Autodesk Inventor part; units mm, degrees
ref_plane "YZ Plane" through (0, 0, 0) normal (1, 0, 0) x (0, 1, 0)
ref_plane "XZ Plane" through (0, 0, 0) normal (0, 1, 0) x (-1, 0, 0)
ref_plane "XY Plane" through (0, 0, 0) normal (0, 0, 1) x (1, 0, 0)
sketch "Sketch1" plane through (0, 0, 0) normal (0, 1, 0) x (-1, 0, 0)
  circle A0 centre (0, 0) radius 11
  circle A1 centre (0, 0) radius 12.5
  dimension "d0" = 22
  dimension "d1" = 25
extrude "Extrusion1" add sketch "Sketch1" along normal blind 7
sketch "Sketch2" plane through (0, 7, 0) normal (0, 1, 0) x (1, 0, 0)
  circle A0 centre (0, -18.05) radius 2.15
  circle A1 centre (0, 18.05) radius 2.15
  circle A2 centre (0, -18.05) radius 5.95
  circle A3 centre (0, 18.05) radius 5.95
  line L0 (-5.5444, -20.2091) -> (-11.6479, -4.536)
  line L1 (5.5444, -20.2091) -> (11.6479, -4.536)
  line L2 (-11.6479, 4.536) -> (-5.5444, 20.2091)
  line L3 (11.6479, 4.536) -> (5.5444, 20.2091)
  circle A4 centre (0, 0) radius 12.5
  dimension "d4" = 4.3
  dimension "d5" = 4.3
  dimension "d6" = 0
  dimension "d7" = 0
  dimension "d8" = 18.05
  dimension "d9" = 18.05
  dimension "d10" = 3.8
  dimension "d11" = 3.8
extrude "Extrusion2" add sketch "Sketch2" against normal blind 3.5 contours A2 A4 | L0 A4 A2 | A2 A4 L1 | L2 A3 A4 | A3 A4 | A4 A3 L3 picked at (3.4679, -21.155) picked at (3.4679, 21.155)
properties part number "chumacera"
Design review of the part built by this model. Coordinates are the model's own, in mm. A direction names the side the tool comes from. Coordinates: 2 decimals unless noted, no trailing zeros. Order: outer loops, then holes, each group sorted by start corner. A loop starts at its lowest first (then second) coordinate and runs counter-clockwise, first axis right, second up.
1) Clearance check with flat-ended pins moving along their axes: pin 1 (5.5 mm diameter, centred on x = 0, z = -18.05, fed in from +Y); pin 2 (2.5 mm diameter, centred on x = 0, z = 18.05, fed in from +Y); pin 3 (3 mm diameter, centred on y = 2.5, z = -7.5, fed in from +X); pin 4 (2 mm diameter, centred on y = 1, z = 9, fed in from -X). State where each tip first meets the part, or that it passes through.
2) Take a section at C-C, the plane x = 9.75. Give the boundary of the cut face in (y, z).
3) Wall thickness on line 1 along Z through (x, y) = (0, 4.75); line 2 along Z through (x, y) = (0, 2); line 3 along X through (y, z) = (3.5, -4): over which ranges is each line inside the solid? List them lowest first.
4) Take a section at A-A, the plane x = 0. Give the boundary of the cut face in (y, z).
5) Take a section at D-D, the plane y = 4.5. Give the boundary of the cut face in (x, z).
6) For faces 1 (the flat face through (-8.553, 5.274, 12.482)), 2 (the cylindrical face through (1.627, 2.673, -12.394)), list the 3-axis set-ups (+Z, -Z, +X, -X, +Y, -Y) from which the entire face can be reached by the end or side of a thin tool; tool diameter is ignored.
7) Take a section at B-B, the plane z = -8. Give the boundary of the cut face in (x, y), and give its area (3 significant figures).
Returned:
1. pin 1: stops at y = 7
1. pin 2: passes through
1. pin 3: stops at x = 10.97
1. pin 4: stops at x = -9.6
2. outline: (0, -7.82) - (3.5, -7.82) - (3.5, -9.41) - (7, -9.41) - (7, -5.09) - (0, -5.09) - close; (0, 5.09) - (7, 5.09) - (7, 9.41) - (3.5, 9.41) - (3.5, 7.82) - (0, 7.82) - close
3. line 1: z = -24 to -20.2, -15.9 to -11, 11 to 15.9, 20.2 to 24
3. line 2: z = -12.5 to -11, 11 to 12.5
3. line 3: x = -11.84 to -10.25, 10.25 to 11.84
4. outline: (0, -12.5) - (3.5, -12.5) - (3.5, -15.9) - (7, -15.9) - (7, -11) - (0, -11) - close; (0, 11) - (7, 11) - (7, 15.9) - (3.5, 15.9) - (3.5, 12.5) - (0, 12.5) - close; (3.5, -24) - (7, -24) - (7, -20.2) - (3.5, -20.2) - close; (3.5, 20.2) - (7, 20.2) - (7, 24) - (3.5, 24) - close
5. outline: (-11.65, -4.54) - (-5.54, -20.21) arc R5.95 ccw to (5.54, -20.21) - (11.65, -4.54) arc R12.5 ccw to (11.65, 4.54) - (5.54, 20.21) arc R5.95 ccw to (-5.54, 20.21) - (-11.65, 4.54) arc R12.5 ccw to start; hole circle Ø22 at (0, 0); hole circle Ø4.3 at (0, -18.05); hole circle Ø4.3 at (0, 18.05)
6. face 1: +Z, -X, +Y, -Y
6. face 2: -Y
7. outline: (-10.3, 3.5) - (-9.6, 3.5) - (-9.6, 0) - (-7.55, 0) - (-7.55, 7) - (-10.3, 7) - close; (7.55, 0) - (9.6, 0) - (9.6, 3.5) - (10.3, 3.5) - (10.3, 7) - (7.55, 7) - close
7. area: 33.6 mm2
